Verification items for the finished model (mm, model axes). Coordinates: 2 decimals unless noted, no trailing zeros. Order: outer loops, then holes, each group sorted by start corner. A loop starts at its lowest first (then second) coordinate and runs counter-clockwise, first axis right, second up. Notation, with made-up numbers: M -36.5,14 L 10.5,14 A14 ccw 10.5,30 Z; hole C 73.25,20.25 d10. An arc over 180 degrees is marked long. Write item = value, one per line.
```python
from build123d import *

# Parameters (mm, degrees)
SKETCH1_W           = 72.5
SKETCH1_H           = 15
BOSS_EXTRUDE1_DEPTH = 1.3
SKETCH2_W           = 1.4
SKETCH2_H           = 10
SKETCH2_W_2         = 20
SKETCH2_H_2         = 1.4
BOSS_EXTRUDE2_DEPTH = 1.3
SKETCH3_W           = 1
SKETCH3_H           = 10
CUT_EXTRUDE1_DEPTH  = 39.709462667
SKETCH4_R           = 3.1
CUT_EXTRUDE2_DEPTH  = 39.709462667


with BuildPart() as part:
    # Sketch1 → Boss-Extrude1 (new body)
    with BuildSketch(Plane(origin=(0, 0, 0), x_dir=(0, 0, -1), z_dir=(1, 0, 0))):
        Rectangle(SKETCH1_W, SKETCH1_H)
    extrude(amount=BOSS_EXTRUDE1_DEPTH)

    # Sketch2 → Boss-Extrude2 (add)
    with BuildSketch(Plane(origin=(1.3, 0, 0), x_dir=(0, 0, -1), z_dir=(1, 0, 0))):
        with Locations((-36.95, 2.5)):
            Rectangle(SKETCH2_W, SKETCH2_H)
        with Locations((36.95, -0.5)):
            Rectangle(SKETCH2_W, SKETCH2_H)
        with Locations((0, -8.2)):
            Rectangle(SKETCH2_W_2, SKETCH2_H_2)
    extrude(amount=-BOSS_EXTRUDE2_DEPTH)

    # Sketch3 → Cut-Extrude1 (cut, through all)
    with BuildSketch(Plane(origin=(1.3, 0, 0), x_dir=(0, 0, -1), z_dir=(1, 0, 0))):
        with Locations((16, 0)):
            Rectangle(SKETCH3_W, SKETCH3_H)
        with Locations((-16, 0)):
            Rectangle(SKETCH3_W, SKETCH3_H)
    extrude(amount=-CUT_EXTRUDE1_DEPTH, mode=Mode.SUBTRACT)

    # Sketch4 → Cut-Extrude2 (cut, through all)
    with BuildSketch(Plane(origin=(1.3, 0, 0), x_dir=(0, 0, -1), z_dir=(1, 0, 0))):
        with Locations((2.75, -3)):
            Circle(SKETCH4_R)
    extrude(amount=-CUT_EXTRUDE2_DEPTH, mode=Mode.SUBTRACT)


solid = part.part
```
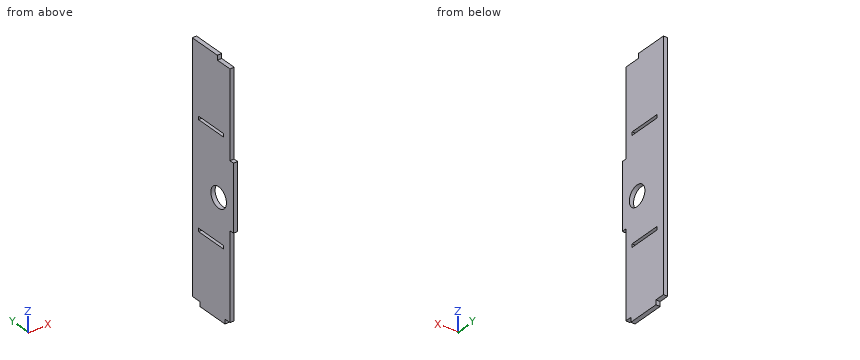
Item 1: Sectioned sample at C-C, the plane y = -0.75. Enter the section's corners in (x, z).
Report:
outline = M 0,-37.65 L 1.3,-37.65 L 1.3,-16.5 L 0,-16.5 Z; M 0,-15.5 L 1.3,-15.5 L 1.3,-4.88 L 0,-4.88 Z; M 0,-0.62 L 1.3,-0.62 L 1.3,15.5 L 0,15.5 Z; M 0,16.5 L 1.3,16.5 L 1.3,37.65 L 0,37.65 Z
Item 2: Sectioned sample at D-D, the plane y = -4. Enter the section's corners in (x, z).
Report:
outline = M 0,-37.65 L 1.3,-37.65 L 1.3,-16.5 L 0,-16.5 Z; M 0,-15.5 L 1.3,-15.5 L 1.3,-5.68 L 0,-5.68 Z; M 0,0.18 L 1.3,0.18 L 1.3,15.5 L 0,15.5 Z; M 0,16.5 L 1.3,16.5 L 1.3,36.25 L 0,36.25 Z
Item 3: Sectioned sample at B-B, the plane x = 0.7. Enter the section's corners in (y, z), then the cut area to 3 significant figures.
Report:
outline = M -8.9,-10 L -7.5,-10 L -7.5,-36.25 L -5.5,-36.25 L -5.5,-37.65 L 4.5,-37.65 L 4.5,-36.25 L 7.5,-36.25 L 7.5,37.65 L -2.5,37.65 L -2.5,36.25 L -7.5,36.25 L -7.5,10 L -8.9,10 Z; hole C -3,-2.75 d6.2; hole M -5,-16.5 L 5,-16.5 L 5,-15.5 L -5,-15.5 Z; hole M -5,15.5 L 5,15.5 L 5,16.5 L -5,16.5 Z
area = 1,090 mm^2
Item 4: Sectioned sample at A-A, the plane z = -2.75. Enter the section's corners in (x, y), then the cut area to 3 significant figures.
Report:
outline = M 0,-8.9 L 1.3,-8.9 L 1.3,-6.1 L 0,-6.1 Z; M 0,0.1 L 1.3,0.1 L 1.3,7.5 L 0,7.5 Z
area = 13.3 mm^2
Item 5: Gauge pin test, flat ends, axial feed: pin 1 (0.6 mm diameter, centred on x = 1, z = -37, fed in from -Y); pin 2 (1 mm diameter, centred on y = -6.5, z = -19, fed in from -X); pin 3 (0.6 mm diameter, centred on x = 1, y = -6.5, fed in from -Z); pin 4 (5.5 mm diameter, centred on y = -3, z = -2.75, fed in from +X). Record the tip position at first contact, or that the pin passes through.
Report:
pin_1 = -5.5
pin_2 = 0
pin_3 = -36.25
pin_4 = through
Item 6: Scan lines: L1, parallel to Z at x = 1.1, y = 1.5; L2, parallel to Z at x = 0.45, y = -1; L3, parallel to Y at x = 0.65, z = -2.75. Record each from-to range of solid material in increasing order. Write a range as from..to.
Report:
L1 = -37.65..-16.5, -15.5..15.5, 16.5..37.65
L2 = -37.65..-16.5, -15.5..-5.12, -0.38..15.5, 16.5..37.65
L3 = -8.9..-6.1, 0.1..7.5
